Could you check a few things on this model? Use its own coordinates, in mm. A direction names the side the tool comes from. Coordinates: 2 decimals unless noted, no trailing zeros. Order: outer loops, then holes, each group sorted by start corner. A loop starts at its lowest first (then second) coordinate and runs counter-clockwise, first axis right, second up. Notation, with made-up numbers: (36, 19.25) - (41, 19.25) arc R27 cw to (41, 36.25) - close; hole circle Ø8 at (36, 66.25). An arc over 180 degrees is marked (long way). Answer as a JSON object with one key per item and string values. Group by question number.
(1) Imagine slicing it at D-D, the plane z = 31.5. Write out the boundary of the cut face in (x, y), and give its area (3 significant figures).
(2) We'd pull the mould along X, two halves only. Please class faces 1 (the flat face through (40, 23, 35)), 2 (the flat face through (37, 8, 43)), 3 (the cylindrical face through (8.17, 4.06, 29.02)): pulls with the +X half, pulls with the -X half, needs draft (parallel to the pull), parting line crosses it, or undercut.
(3) Will these pins go through, and if not, where does the flat tip stop? P1, Ø0.5, axis at y = 4.5, z = 47, coming from the +X side; P2, Ø3, axis at x = 35, y = 18, coming from the -Z side; P3, Ø0.8, axis at x = -32.5, z = 47, coming from the -Y side; P4, Ø4, axis at y = 11, z = 4.5, coming from the -X side.
(4) Imagine slicing it at B-B, the plane z = -19. Write out the boundary of the cut face in (x, y).
(5) Imagine slicing it at C-C, the plane y = 4. Write out the boundary of the cut face in (x, z).
(6) Please list where these lines run through material, in increasing order: probe 1 along X at (y, z) = (4.5, 31.5); probe 2 along X at (y, z) = (2, 31); probe 3 along Y at (x, z) = (37, -30.5).
(7) Which directions (+Z, -Z, +X, -X, +Y, -Y) give clear straight access to the entire face, cutting with the end or side of a thin tool? Please do faces 4 (the flat face through (36.87, 22.79, 41.92)), 5 (the flat face through (-38, 8, 44)), 6 (the flat face through (-35, 23, 33.5)), 7 (the flat face through (-30.649, 23, 41)), 8 (the flat face through (32, 23, 47.5)).
(8) Imagine slicing it at A-A, the plane x = 8.5. Write out the boundary of the cut face in (y, z).
Autodesk Inventor part; units mm, degrees
ref_plane "YZ Plane" through (0, 0, 0) normal (1, 0, 0) x (0, 1, 0)
ref_plane "XZ Plane" through (0, 0, 0) normal (0, 1, 0) x (-1, 0, 0)
ref_plane "XY Plane" through (0, 0, 0) normal (0, 0, 1) x (1, 0, 0)
sketch "Sketch1" plane through (0, 0, 0) normal (0, 1, 0) x (-1, 0, 0)
  line L0 (40, 47.5) -> (-40, 47.5)
  line L1 (-40, 47.5) -> (-40, -47.5)
  line L2 (-40, -47.5) -> (40, -47.5)
  line L3 (40, -47.5) -> (40, 47.5)
  line L4 (40, 47.5) -> (-40, -47.5) construction
  line L5 (-40, 47.5) -> (40, -47.5) construction
  point P0 (0, 0)
  dimension "d0" = 80
  dimension "d1" = 95
extrude "Extrusion1" add sketch "Sketch1" along normal blind 8
sketch "Sketch2" plane through (0, 8, 0) normal (0, 1, 0) x (1, 0, 0)
  line L0 (0, 0) -> (0, 19)
  line L1 (0, 19) -> (24, 19)
  line L2 (0, 0) -> (0, -31.5)
  line L3 (0, -31.5) -> (-19.5, -31.5)
  line L4 (0, -31.5) -> (8.5, -31.5)
  circle A0 centre (8.5, -31.5) radius 2.5
  circle A1 centre (-19.5, -31.5) radius 2.5
  circle A2 centre (24, 19) radius 2.5
  dimension "d4" = 19
  dimension "d5" = 24
  dimension "d6" = 31.5
  dimension "d7" = 19.5
  dimension "d8" = 8.5
  dimension "d9" = 5
  dimension "d10" = 5
  dimension "d11" = 5
extrude "Extrusion2" cut sketch "Sketch2" against normal blind 8
sketch "Sketch4" plane through (0, 8, 0) normal (0, 1, 0) x (1, 0, 0)
  line L0 (-40, -47.5) -> (40, -47.5)
  line L1 (-40, -47.5) -> (-40, -36.5)
  line L2 (-40, -36.5) -> (-33.6491, -47.5)
  line L3 (-33.6491, -47.5) -> (-30.6491, -47.5)
  line L4 (-30.6491, -47.5) -> (-30.6491, -33.5)
  line L5 (-30.6491, -33.5) -> (-40, -33.5)
  line L6 (-40, 47.5) -> (-40, -47.5)
  line L7 (-40, -36.5) -> (-40, -33.5)
  line L8 (0, -20.8898) -> (0, -30.7247)
  line L9 (40, -47.5) -> (40, -36.5)
  line L10 (40, -36.5) -> (33.6491, -47.5)
  line L11 (33.6491, -47.5) -> (30.6491, -47.5)
  line L12 (30.6491, -47.5) -> (30.6491, -33.5)
  line L13 (30.6491, -33.5) -> (40, -33.5)
  line L14 (40, -36.5) -> (40, -33.5)
  point P0 (0, 0)
  point P1 (-32.5008, -49.4891)
  point P2 (32.5008, -49.4891)
  dimension "d14" = 11
  dimension "d15" = 30
  dimension "d16" = 3
  dimension "d17" = 14
extrude "Extrusion3" add sketch "Sketch4" along normal blind 30 contours L12 L13 L14 L10 L0 | L2 L6 L5 L4 L0
sketch "Sketch5" plane through (0, 0, 0) normal (0, -1, 0) x (1, 0, 0)
  circle A0 centre (-19.5, 31.5) radius 2.5
  circle A1 centre (8.5, 31.5) radius 2.5
  circle A2 centre (24, -19) radius 2.5
  line L0 (-40, 47.5) -> (40, 47.5)
  line L1 (-40, -47.5) -> (-40, 47.5)
  line L2 (40, -47.5) -> (-40, -47.5)
  line L3 (40, 47.5) -> (40, -47.5)
  line L4 (40, 47.5) -> (40, -12.5)
  line L5 (40, -12.5) -> (39, -12.5)
  line L6 (39, -12.5) -> (39, 47.5)
  line L7 (33.6491, 47.5) -> (40, 47.5)
  line L8 (40, 47.5) -> (39, 47.5)
  line L9 (40, 47.5) -> (40, 46.5)
  line L10 (40, 47.5) -> (40, 36.5)
  line L11 (40, 46.5) -> (30, 46.5)
  line L12 (30, 46.5) -> (30, 47.5)
  line L13 (40, 47.5) -> (30, 47.5)
  line L14 (-30.6491, 47.5) -> (30.6491, 47.5)
  line L15 (0, 47.5) -> (0, 0)
  line L16 (-40, 47.5) -> (-40, -12.5)
  line L17 (-40, -12.5) -> (-39, -12.5)
  line L18 (-39, -12.5) -> (-39, 47.5)
  line L19 (-33.6491, 47.5) -> (-40, 47.5)
  line L20 (-40, 47.5) -> (-39, 47.5)
  line L21 (-40, 47.5) -> (-40, 46.5)
  line L22 (-40, 47.5) -> (-40, 36.5)
  line L23 (-40, 46.5) -> (-30, 46.5)
  line L24 (-30, 46.5) -> (-30, 47.5)
  line L25 (-40, 47.5) -> (-30, 47.5)
  dimension "d20" = 60
  dimension "d21" = 1
  dimension "d22" = 1
  dimension "d23" = 10
extrude "Extrusion4" cut sketch "Sketch5" against normal blind 8 contours L0 L18 L23 L1 | L0 L24 L23 L18 | L23 L18 L17 L1 | L0 L6 L11 L12 | L5 L6 L11 L3 | L6 L0 L3 L11
properties part number "Base"
Result set:
{
 "1": {"outline": "(-39, 0) - (-22, 0) - (-22, 8) - (-39, 8) - close; (-17, 0) - (6, 0) - (6, 8) - (-17, 8) - close; (11, 0) - (39, 0) - (39, 8) - (11, 8) - close", "area": "544 mm^2"},
 "2": {"face 1": "pulls with the +X half", "face 2": "needs draft", "face 3": "undercut"},
 "3": {"P1": "stops at x = 30", "P2": "stops at z = 33.5", "P3": "stops at y = 8", "P4": "passes through"},
 "4": {"outline": "(-40, 0) - (21.5, 0) - (21.5, 8) - (-40, 8) - close; (26.5, 0) - (40, 0) - (40, 8) - (26.5, 8) - close"},
 "5": {"outline": "(-40, -47.5) - (40, -47.5) - (40, -12.5) - (39, -12.5) - (39, 46.5) - (30, 46.5) - (30, 47.5) - (-30, 47.5) - (-30, 46.5) - (-39, 46.5) - (-39, -12.5) - (-40, -12.5) - close; hole circle Ø5 at (-19.5, 31.5); hole circle Ø5 at (8.5, 31.5); hole circle Ø5 at (24, -19)"},
 "6": {"probe 1": "x = -39 to -22, -17 to 6, 11 to 39", "probe 2": "x = -39 to -21.95, -17.05 to 6.05, 10.95 to 39", "probe 3": "y = 0 to 8"},
 "7": {"face 4": "+Z, +X, +Y", "face 5": "+Z, -X, +Y", "face 6": "-Z, +X, -X, +Y", "face 7": "+Z, -Z, +Y", "face 8": "+Z, +X, -X, +Y, -Y"},
 "8": {"outline": "(0, -47.5) - (8, -47.5) - (8, 29) - (0, 29) - close; (0, 34) - (8, 34) - (8, 47.5) - (0, 47.5) - close"}
}
